```python
from build123d import *

# Parameters (mm, degrees)
F0_W     = 3.2
F0_H     = 6.1
F0_R     = 2.5
F0_W_2   = 7
F0_H_2   = 3.2
F0_W_3   = 33.5989631712
F0_H_3   = 26.0656554639
F0_W_4   = 8
F0_R_2   = 5.5
F1_DEPTH = 1.5


with BuildPart() as f1:
    # F0 (on Top) → F1 (new body, symmetric)
    with BuildSketch(Plane.XY):
        with BuildLine():
            Line((0, 49.5), (-31, 37.5))
            add(Edge.make_bspline(
                [(-31, 37.5), (-38.1511552694, 25.7567925156), (-53.9932959403, -0.2582411241), (-39.1454927008, -37.415537584), (-31, -57.8)],
                knots=[0, 0, 0, 0, 0.4514008187, 1, 1, 1, 1], degree=3))
            Line((-31, -57.8), (0, -69.8))
            Line((0, -69.8), (31, -57.8))
            add(Edge.make_bspline(
                [(31, 37.5), (38.1511552694, 25.7567925156), (53.9932959403, -0.2582411241), (39.1454927008, -37.415537584), (31, -57.8)],
                knots=[0, 0, 0, 0, 0.4514008187, 1, 1, 1, 1], degree=3))
            Line((31, 37.5), (0, 49.5))
        make_face()
        with Locations((-27.1, -43.65)):
            Rectangle(F0_W, F0_H, mode=Mode.SUBTRACT)
        Polygon((-20, -45.92561), (-20, -50.12561), (-20, -51.42561), (-23.2, -51.42561), (-23.2, -50.12561), (-23.2, -45.92561), align=None, mode=Mode.SUBTRACT)
        Polygon((-20, -37.52561), (-20, -41.72561), (-20, -42.5726920366), (-23.2, -42.5726920366), (-23.2, -41.72561), (-23.2, -37.52561), align=None, mode=Mode.SUBTRACT)
        with Locations((-27.1, -31.45)):
            Rectangle(F0_W, F0_H, mode=Mode.SUBTRACT)
        Polygon((-20, -29.12561), (-20, -33.32561), (-20, -34.545276314), (-23.2, -34.545276314), (-23.2, -33.32561), (-23.2, -29.12561), align=None, mode=Mode.SUBTRACT)
        with Locations((-24.5, -24)):
            Circle(F0_R, mode=Mode.SUBTRACT)
        with Locations((-6.5, -20.9)):
            Rectangle(F0_W_2, F0_H_2, mode=Mode.SUBTRACT)
        Polygon((0, -66.37), (-22.14, -57.8), (-14, -57.8), (-14, -54.6), (-7, -54.6), (-7, -57.8), (0, -57.8), (0, -54.6), (7, -54.6), (7, -57.8), (14, -57.8), (14, -54.6), (21, -54.6), (21, -57.8), (22.14, -57.8), align=None, mode=Mode.SUBTRACT)
        Polygon((20, -50.12561), (20, -45.92561), (23.2, -45.92561), (23.2, -50.12561), (23.2, -51.42561), (20, -51.42561), align=None, mode=Mode.SUBTRACT)
        Polygon((20, -37.52561), (23.2, -37.52561), (23.2, -41.72561), (23.2, -42.5726920366), (20, -42.5726920366), (20, -41.72561), align=None, mode=Mode.SUBTRACT)
        with Locations((27.1, -43.65)):
            Rectangle(F0_W, F0_H, mode=Mode.SUBTRACT)
        with Locations((0, -37.95)):
            Rectangle(F0_W_3, F0_H_3, mode=Mode.SUBTRACT)
        Polygon((20, -29.12561), (23.2, -29.12561), (23.2, -33.32561), (23.2, -34.545276314), (20, -34.545276314), (20, -33.32561), align=None, mode=Mode.SUBTRACT)
        with Locations((6.5, -20.9)):
            Rectangle(F0_W_2, F0_H_2, mode=Mode.SUBTRACT)
        with Locations((24.5, -24)):
            Circle(F0_R, mode=Mode.SUBTRACT)
        with Locations((27.1, -31.45)):
            Rectangle(F0_W, F0_H, mode=Mode.SUBTRACT)
        with BuildLine():
            Line((-31, -22.5), (-31, -32.5))
            Line((-31, -32.5), (-31, -50.3))
            add(Edge.make_bspline(
                [(-31, 32.5), (-36.6370197512, 22.3171385617), (-49.1609689327, -0.3064541885), (-37.4434647152, -32.5624194988), (-31, -50.3)],
                knots=[0, 0, 0, 0, 0.4500992195, 1, 1, 1, 1], degree=3))
            Line((-31, 32.5), (-31, 22.5))
            Line((-31, 22.5), (-27.8, 22.5))
            Line((-27.8, 22.5), (-27.8, 7.5))
            Line((-27.8, 7.5), (-31, 7.5))
            Line((-31, 7.5), (-31, -7.5))
            Line((-31, -7.5), (-27.8, -7.5))
            Line((-27.8, -7.5), (-27.8, -22.5))
            Line((-27.8, -22.5), (-31, -22.5))
        make_face(mode=Mode.SUBTRACT)
        with Locations((-20.4, -7.8)):
            Rectangle(F0_W, F0_H_2, mode=Mode.SUBTRACT)
        with Locations((-14, -7.8)):
            Rectangle(F0_W, F0_H_2, mode=Mode.SUBTRACT)
        with Locations((-7.6, -7.8)):
            Rectangle(F0_W, F0_H_2, mode=Mode.SUBTRACT)
        with Locations((-20.4, 7.8)):
            Rectangle(F0_W, F0_H_2, mode=Mode.SUBTRACT)
        with Locations((-14, 7.8)):
            Rectangle(F0_W, F0_H_2, mode=Mode.SUBTRACT)
        with Locations((-7.6, 7.8)):
            Rectangle(F0_W, F0_H_2, mode=Mode.SUBTRACT)
        with Locations((-24.5, 34)):
            Circle(F0_R, mode=Mode.SUBTRACT)
        with Locations((-17, 29.6)):
            Rectangle(F0_W_4, F0_H_2, mode=Mode.SUBTRACT)
        with Locations((-1, 29.6)):
            Rectangle(F0_W_4, F0_H_2, mode=Mode.SUBTRACT)
        with Locations((7.6, -7.8)):
            Rectangle(F0_W, F0_H_2, mode=Mode.SUBTRACT)
        Circle(F0_R_2, mode=Mode.SUBTRACT)
        with Locations((14, -7.8)):
            Rectangle(F0_W, F0_H_2, mode=Mode.SUBTRACT)
        with Locations((20.4, -7.8)):
            Rectangle(F0_W, F0_H_2, mode=Mode.SUBTRACT)
        with Locations((7.6, 7.8)):
            Rectangle(F0_W, F0_H_2, mode=Mode.SUBTRACT)
        with Locations((14, 7.8)):
            Rectangle(F0_W, F0_H_2, mode=Mode.SUBTRACT)
        with Locations((20.4, 7.8)):
            Rectangle(F0_W, F0_H_2, mode=Mode.SUBTRACT)
        with BuildLine():
            Line((27.8, 7.5), (27.8, 22.5))
            Line((27.8, 22.5), (31, 22.5))
            Line((31, 22.5), (31, 32.5))
            add(Edge.make_bspline(
                [(31, 32.5), (36.6370197512, 22.3171385617), (49.1609689327, -0.3064541885), (37.4434647152, -32.5624194988), (31, -50.3)],
                knots=[0, 0, 0, 0, 0.4500992195, 1, 1, 1, 1], degree=3))
            Line((31, -50.3), (31, -32.5))
            Line((31, -32.5), (31, -22.5))
            Line((31, -22.5), (27.8, -22.5))
            Line((27.8, -22.5), (27.8, -7.5))
            Line((27.8, -7.5), (31, -7.5))
            Line((31, -7.5), (31, 7.5))
            Line((31, 7.5), (27.8, 7.5))
        make_face(mode=Mode.SUBTRACT)
        with Locations((15, 29.6)):
            Rectangle(F0_W_4, F0_H_2, mode=Mode.SUBTRACT)
        with Locations((24.5, 34)):
            Circle(F0_R, mode=Mode.SUBTRACT)
        Polygon((22.1355892594, 37.5), (0, 37.5), (-22.1355892594, 37.5), (0, 46.0686151972), align=None, mode=Mode.SUBTRACT)
    extrude(amount=F1_DEPTH, both=True)


solid = f1.part
```
Could you check a few things on this model? Use its own coordinates, in mm. Coordinates: 2 decimals unless noted, no trailing zeros. Return JSON: item names as keys, results as strings.
(1) I'm going to push flat-ended pins straight in: pin 1 (3 mm diameter, centred on x = 2, y = -27, fed in from +Z); pin 2 (0.9 mm diameter, centred on y = -41, z = -0.5, fed in from +X); pin 3 (1.5 mm diameter, centred on y = -8, z = 0.5, fed in from -X); pin 4 (0.9 mm diameter, centred on x = 5, z = -0.5, fed in from -Y). Where does each tip first touch, or does it pass through?
Numbers:
{"pin 1": "passes through", "pin 2": "stops at x = 37.71", "pin 3": "stops at x = -46.15", "pin 4": "stops at y = -68.04"}
(2) Imagine slicing it at A-A, the plane y = 0. Count the separate pieces of the cut face and the enclosed holes in it, then the cut area to 3 significant figures.
Numbers:
{"separate pieces": "4", "enclosed holes": "0", "area": "172 mm2"}
(3) I need wall thicknesses on L1, parallel to Y at x = 24.5, z = 0.55; L2, parallel to Y at x = -11.5, z = -0.1; L3, parallel to X at y = -28.5, z = 0.5. Which ranges of each line are inside material? Lowest first, please.
Numbers:
{"L1": "y = -60.32 to -26.5, -21.5 to 31.5, 36.5 to 40.02", "L2": "y = -65.35 to -61.92, -54.6 to -50.98, -24.92 to 37.5, 41.62 to 45.05", "L3": "x = -41.81 to -38.48, -31 to -28.7, -25.5 to -16.8, 16.8 to 25.5, 28.7 to 31, 38.48 to 41.81"}
(4) We'd pull the mould along Y, two halves only. Please class faces 1 (the flat face through (-29, 7.5, 0)), 2 (the flat face through (15.283, -63.884, 0.021)), 3 (the flat face through (4, -5, 1.5)), 4 (the flat face through (15.717, 43.416, 0.021)): +Y half, -Y half, draft (parallel to the pull), parting line (faces both ways), or undercut.
Numbers:
{"face 1": "undercut", "face 2": "-Y half", "face 3": "draft", "face 4": "+Y half"}
